```python
from build123d import *

# Parameters (mm, degrees)
BOSS_EXTRUDE1_DEPTH = 25
SKETCH2_R           = 2.5
CUT_EXTRUDE1_DEPTH  = 68


with BuildPart() as part:
    # Sketch1 → Boss-Extrude1 (new body)
    with BuildSketch(Plane(origin=(0, 0, 0), x_dir=(1, 0, 0), z_dir=(0, 1, 0))):
        Polygon((0, 0), (20, 0), (20, -3), (0, -3), (0, -55), (-18, -55), (-48, -55), (-48, -52), (-3, -52), (-3, 0), align=None)
    extrude(amount=BOSS_EXTRUDE1_DEPTH)

    # Sketch2 → Cut-Extrude1 (cut)
    with BuildSketch(Plane.XY.offset(55)):
        with Locations((-40, 12.5)):
            Circle(SKETCH2_R)
        with Locations((10, 12.5)):
            Circle(SKETCH2_R)
    extrude(amount=-CUT_EXTRUDE1_DEPTH, mode=Mode.SUBTRACT)


solid = part.part
```
Could you check a few things on this model? Use its own coordinates, in mm. A direction names the side the tool comes from. Give positions to 0.01 mm unless a question says otherwise; leave off trailing zeros. Order: outer loops, then holes, each group sorted by start corner. A loop starts at its lowest first (then second) coordinate and runs counter-clockwise, first axis right, second up.
Q1. Suppose I cut it at B-B, the plane x = 10. Write out the boundary of the cut face in (y, z).
Q2. We'd pull the mould along Y, two halves only. Please class faces 4 (the flat face through (-1, 25, 29)), 5 (the flat face through (-1, 0, 29)), 6 (the cylindrical face through (-37.69, 11.54, 53.52)): +Y half, -Y half, draft (parallel to the pull), parting line (faces both ways), or undercut.
Q3. Suppose I cut it at D-D, the plane z = 21. Write out the boundary of the cut face in (x, y).
Q4. Suppose I cut it at A-A, the plane y = 12.5. Write out the boundary of the cut face in (x, z), and give its area (3 significant figures).
Q5. Suppose I cut it at C-C, the plane y = 20. Write out the boundary of the cut face in (x, z).
Q6. I'm going to push flat-ended pins straight in: P1, Ø12.5, axis at y = 16.5, z = 20, coming from the +X side; P2, Ø10, axis at x = -4.5, z = 14, coming from the -Y side; P3, Ø12.5, axis at y = 18, z = 30.5, coming from the -X side; P4, Ø4, axis at x = -6.5, z = 20, coming from the +Y side. Where does each tip first touch, or does it pass through?
Q7. For faces 1 (the flat face through (-26, 12, 52)), 2 (the flat face through (0, 12, 29)), 3 (the flat face through (-24, 12, 55)), which set-ups out of +Z, -Z, +X, -X, +Y, -Y let a thin tool reach every point of the face, with its end or its side?
Q8. If I drill on line 1 along Y through (x, z) = (-40, 53.1); line 2 along Z through (x, y) = (-29, 18.75); line 3 along Z through (x, y) = (0.5, 20.5), over which ranges is the centre line in solid material (lowest first)?
Solution:
1. outline: (0, 0) - (10, 0) - (10, 3) - (0, 3) - close; (15, 0) - (25, 0) - (25, 3) - (15, 3) - close
2. face 4: +Y half
2. face 5: -Y half
2. face 6: undercut
3. outline: (-3, 0) - (0, 0) - (0, 25) - (-3, 25) - close
4. outline: (-48, 52) - (-42.5, 52) - (-42.5, 55) - (-48, 55) - close; (-37.5, 52) - (-3, 52) - (-3, 0) - (7.5, 0) - (7.5, 3) - (0, 3) - (0, 55) - (-37.5, 55) - close; (12.5, 0) - (20, 0) - (20, 3) - (12.5, 3) - close
4. area: 330 mm2
5. outline: (-48, 52) - (-3, 52) - (-3, 0) - (20, 0) - (20, 3) - (0, 3) - (0, 55) - (-48, 55) - close
6. P1: stops at x = 0
6. P2: stops at y = 0
6. P3: stops at x = -3
6. P4: passes through
7. face 1: -Z, -X, +Y, -Y
7. face 2: +Z, +X, +Y, -Y
7. face 3: +Z, +X, -X, +Y, -Y
8. line 1: y = 0 to 10, 15 to 25
8. line 2: z = 52 to 55
8. line 3: z = 0 to 3
